Source: CAD feature listing. Evaluate the final solid. Frame: model axes, mm. A direction names the side the tool comes from. Round coordinates to 2 decimals unless told otherwise and drop trailing zeros. Loops run counter-clockwise (first coordinate to the right, second up) from the corner with the lowest first, then second, coordinate; pieces in that order, holes last. Notation, with made-up numbers: M 81,15.5 L 136,15.5 A33 ccw 136,51.5 Z; hole C 70,28 d11. An arc over 180 degrees is marked long. Answer as CSV lines item,"result". Start each with the question number.
```python
from build123d import *

# Parameters (mm, degrees)
F0_W      = 117.3750758171
F0_H      = 69.6533750743
F1_DEPTH  = 50.8
F3_DEPTH  = 25.4
F4_DEPTH  = 82.804
F6_DEPTH  = 25.4
F8_R      = 10.3010134133
F9_DEPTH  = 146.558
F7_R      = 11.2481723065
F10_DEPTH = 101.6


with BuildPart() as f1:
    # F0 (on Top) → F1 (new body)
    with BuildSketch(Plane.XY):
        with Locations((14.7226527333, 5.685989745)):
            Rectangle(F0_W, F0_H)
    extrude(amount=F1_DEPTH)

    # F2 (on face) → F3 (join)
    with BuildSketch(Plane.XZ.offset(29.1406977922)):
        with BuildLine():
            Line((2.0829490386, 50.8), (-10.5567546561, 50.8))
            ThreePointArc((-10.5567546561, 50.8), (14.8472036235, 35.3357176843), (40.2511619031, 50.8))
            Line((40.2511619031, 50.8), (27.4869073182, 50.8))
            ThreePointArc((27.4869073182, 50.8), (14.7849281784, 42.4531644715), (2.0829490386, 50.8))
        make_face()
    extrude(amount=F3_DEPTH)

    # F4 (cut): a face of the model
    f4_faces = [f1.faces().sort_by_distance(p)[0] for p in [
        (14.7849281784, -29.1406977922, 47.3563909232),
    ]]
    extrude(f4_faces, amount=-F4_DEPTH, mode=Mode.SUBTRACT)

    # F5 (on face) → F6 (join)
    with BuildSketch(Plane(origin=(0, 40.5126772821, 0), x_dir=(-1, 0, 0), z_dir=(0, 1, 0))):
        with BuildLine():
            ThreePointArc((-2.0829490386, 50.8), (-14.7849281784, 42.4531644715), (-27.4869073182, 50.8))
            Line((-27.4869073182, 50.8), (-40.1620790362, 50.8))
            ThreePointArc((-40.1620790362, 50.8), (-14.7955128923, 33.6886739467), (10.5710532516, 50.8))
            Line((10.5710532516, 50.8), (-2.0829490386, 50.8))
        make_face()
    extrude(amount=F6_DEPTH)

    # F8 (on face) → F9 (cut)
    with BuildSketch(Plane.XY.offset(50.8)):
        with Locations((54.6979308128, 3.0329860747)):
            Circle(F8_R)
    extrude(amount=-F9_DEPTH, mode=Mode.SUBTRACT)

    # F7 (on face) → F10 (cut)
    with BuildSketch(Plane.XY.offset(50.8)):
        with Locations((-20.6904988736, 4.6597607434)):
            Circle(F7_R)
    extrude(amount=-F10_DEPTH, mode=Mode.SUBTRACT)


solid = f1.part
```
1) Section A-A, the plane x = 56.5. Return loops of the section in (y, z), and give its area (3 significant figures).
2) Mould query, pull axis Y, two halves, no side actions, for faces 1 (the flat face through (14, 40.513, 25)), 2 (the cylindrical face through (-31.928, 5.154, 25.756)), 3 (the cylindrical face through (64.523, 6.127, 25.756)), 4 (the cylindrical face through (14.41, -41.66, 35.34)). Classes: pulls with the +Y half, pulls with the -Y half, needs draft (parallel to the pull), parting line crosses it, or undercut.
3) Contact query for flat-ended pins moving along their axis: pin 1 Ø2 at (x, z) = (53.5, 22.5) entering from +Y; pin 2 Ø15 at (x, z) = (10.5, 15.5) entering from -Y; pin 3 Ø5 at (x, y) = (21.5, 41.5) entering from +Z; pin 4 Ø18 at (x, y) = (-20.69, 4.66) entering from +Z. Output: stop coordinate, or through.
4) Section B-B, the plane z = 39.5. Return loops of the section in (x, y).
5) Section D-D, the plane z = 10. Return loops of the section in (x, y), and give its area (3 significant figures).
6) Section C-C, the plane y = 55. Return loops of the section in (x, z), and give its area (3 significant figures).
7) Ray query, line 1 along X through (y, z) = (9, 32.5); line 2 along Y through (x, z) = (68.5, 11.5); line 3 along X through (y, z) = (6, 18.5). Return the intervals inside material, ascending.
8) Access query for faces 5 (the flat face through (73.41, 5, 25)), 6 (the cylindrical face through (15.25, 53.035, 33.692)), 7 (the flat face through (14, -29.141, 25)). Directions: +Z, -Z, +X, -X, +Y, -Y. A direction counts if a zero-diameter tool reaches every point of the face in a straight line with its end or side. Return the directions, or none.
Findings below:
1,outline,"M -29.14,0 L -7.11,0 L -7.11,50.8 L -29.14,50.8 Z; M 13.18,0 L 40.51,0 L 40.51,50.8 L 13.18,50.8 Z"
1,area,"2,510 mm²"
2,face 1,"pulls with the +Y half"
2,face 2,"undercut"
2,face 3,"undercut"
2,face 4,"needs draft"
3,pin 1,"y = 40.51"
3,pin 2,"y = -29.14"
3,pin 3,"z = 45.97"
3,pin 4,"through"
4,outline,"M -43.96,-29.14 L -0.01,-29.14 L -0.01,-54.54 L 29.71,-54.54 L 29.71,-29.14 L 73.41,-29.14 L 73.41,40.51 L 31.65,40.51 L 31.65,65.91 L -2.06,65.91 L -2.06,40.51 L -43.96,40.51 Z; hole C -20.69,4.66 d22.5; hole C 54.7,3.03 d20.6"
5,outline,"M -43.96,-29.14 L 73.41,-29.14 L 73.41,40.51 L -43.96,40.51 Z; hole C -20.69,4.66 d22.5; hole C 54.7,3.03 d20.6"
5,area,"7,440 mm²"
6,outline,"M -10.57,50.8 A27.36 ccw 40.16,50.8 L 27.49,50.8 A13.84 cw 2.08,50.8 Z"
6,area,"476 mm²"
7,line 1,"-43.96 to -31.07, -10.31 to 46.3, 63.09 to 73.41"
7,line 2,"-29.14 to 40.51"
7,line 3,"-43.96 to -31.86, -9.52 to 44.83, 64.56 to 73.41"
8,face 5,"+Z, -Z, +X, +Y, -Y"
8,face 6,"-Z, +Y"
8,face 7,"-Z, -Y"
